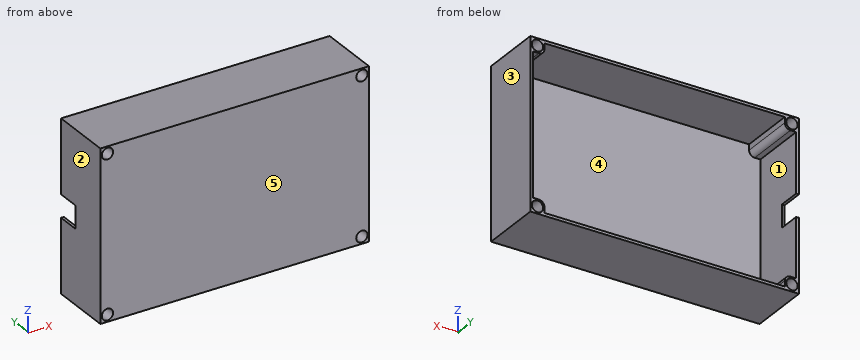
Autodesk Inventor part; units mm, degrees
ref_plane "YZ Plane" through (0, 0, 0) normal (1, 0, 0) x (0, 1, 0)
ref_plane "XZ Plane" through (0, 0, 0) normal (0, 1, 0) x (-1, 0, 0)
ref_plane "XY Plane" through (0, 0, 0) normal (0, 0, 1) x (1, 0, 0)
sketch "Szkic1" plane through (0, 0, 0) normal (0, 1, 0) x (-1, 0, 0)
  line L0 (0, 0) -> (90, 0)
  line L1 (90, 0) -> (90, -60)
  line L2 (90, -60) -> (0, -60)
  line L3 (0, -60) -> (0, 0)
  dimension "d0" = 90
  dimension "d1" = 60
extrude "Wyciągnięcie proste1" add sketch "Szkic1" along normal blind 2
sketch "Szkic15" plane through (-90, 0, -60) normal (-1, 0, 0) x (0, 0, 1)
  line L0 (0, 0) -> (60, 0)
  line L1 (60, 0) -> (60, 2)
  line L2 (60, 2) -> (0, 2)
  line L3 (0, 2) -> (0, 0)
extrude "Wyciągnięcie proste5" add sketch "Szkic15" along normal blind 5
sketch "Szkic16" plane through (0, 2, 0) normal (0, 1, 0) x (1, 0, 0)
  line L0 (0, 60) -> (-95, 60)
  line L1 (-95, 60) -> (-95, 0)
  line L2 (-94, 60) -> (-95, 60)
  line L3 (-95, 60) -> (-95, 0)
  line L4 (-95, 0) -> (-94, 0)
  line L5 (-94, 0) -> (-94, 60)
  line L6 (-95, 1) -> (0, 1)
  line L7 (0, 1) -> (0, 0)
  line L8 (0, 0) -> (-95, 0)
  line L9 (-95, 0) -> (-95, 1)
  line L10 (-1, 0) -> (0, 0)
  line L11 (0, 0) -> (0, 60)
  line L12 (0, 60) -> (-1, 60)
  line L13 (-1, 60) -> (-1, 0)
  line L14 (-1, 59) -> (-95, 59)
  line L15 (-95, 59) -> (-95, 60)
  line L16 (-95, 60) -> (-1, 60)
  line L17 (-1, 60) -> (-1, 59)
  point P0 (-94, 59)
  point P1 (-1, 1)
  point P2 (-94, 1)
extrude "Wyciągnięcie proste6" add sketch "Szkic16" along normal blind 20 contours L11 L6 L13 L0 | L13 L14 L5 L0 | L7 L8 L13 L6 | L5 L14 L1 L0 | L13 L8 L5 L6 | L5 L6 L1 L14 | L5 L4 L1 L6
sketch "Szkic21" plane through (0, 2, 0) normal (0, 1, 0) x (1, 0, 0)
  line L0 (-1, 59) -> (-1, 1)
  line L1 (-94, 1) -> (-1, 1)
  line L2 (-1, 5) -> (-5, 5)
  line L3 (-5, 5) -> (-5, 1)
  line L4 (-5, 1) -> (-1, 1)
  line L5 (-1, 1) -> (-1, 5)
  point P0 (0, 0)
  dimension "d61" = 4
extrude "Wyciągnięcie proste8" add sketch "Szkic21" along normal blind 20
sketch "Szkic22" plane through (0, 2, 0) normal (0, 1, 0) x (1, 0, 0)
  line L0 (-1, 59) -> (-1, 1)
  line L1 (-1, 55) -> (-5, 55)
  line L2 (-5, 55) -> (-5, 59)
  line L3 (-5, 59) -> (-1, 59)
  line L4 (-1, 59) -> (-1, 55)
  line L5 (-94, 1) -> (-94, 59)
  line L6 (-1, 59) -> (-94, 59)
  line L7 (-94, 55) -> (-90, 55)
  line L8 (-90, 55) -> (-90, 59)
  line L9 (-90, 59) -> (-94, 59)
  line L10 (-94, 59) -> (-94, 55)
  line L11 (-94, 1) -> (-5, 1)
  line L12 (-94, 5) -> (-90, 5)
  line L13 (-90, 5) -> (-90, 1)
  line L14 (-90, 1) -> (-94, 1)
  line L15 (-94, 1) -> (-94, 5)
  point P0 (0, 0)
  point P1 (-1, 5)
  dimension "d64" = 4
  dimension "d65" = 4
extrude "Wyciągnięcie proste9" add sketch "Szkic22" along normal blind 20
fillet "Zaokrąglenie1" radius 2 4 edges at (-90, 12, -55) (-5, 12, -55) (-90, 12, -5) (-5, 12, -5)
sketch "Szkic23" plane through (0, 22, 0) normal (0, 1, 0) x (1, 0, 0)
  point P0 (0, 0)
  point P1 (-2.5, 2.5)
  point P2 (-92.5, 2.5)
  point P3 (-92.5, 57.5)
  point P4 (-2.5, 57.5)
hole "Otwór5" at (-2.5, 22, -2.5) at (-92.5, 22, -2.5) at (-92.5, 22, -57.5) at (-2.5, 22, -57.5) direction (0, -1, 0) diameter 4 end through all
sketch "Szkic24" plane through (-95, 0, -60) normal (-1, 0, 0) x (0, 0, 1)
  point P0 (60, 0)
sketch "Szkic25" plane through (-95, 0, 0) normal (0, 0, 1) x (1, 0, 0)
  point P0 (95, 0)
sketch "Szkic26" plane through (-95, 0, -60) normal (-1, 0, 0) x (0, 0, 1)
  line L0 (60, 22) -> (0, 22)
  line L1 (26, 22) -> (34, 22)
  line L2 (34, 22) -> (34, 14)
  line L3 (34, 14) -> (26, 14)
  line L4 (26, 14) -> (26, 22)
  point P0 (60, 0)
  dimension "d76" = 8
  dimension "d77" = 8
extrude "Wyciągnięcie proste10" cut sketch "Szkic26" against normal blind 10
properties part number "góra"
Geometry: final body of the model. Coordinates: model frame, mm. Face numbers are marked on the shaded views. A direction names the side the tool comes from. Round coordinates to 2 decimals unless told otherwise and drop trailing zeros. Loops run counter-clockwise (first coordinate to the right, second up) from the corner with the lowest first, then second, coordinate; pieces in that order, holes last. Notation, with made-up numbers: (80, -12) -> (131, -12) arc R30 ccw to (131, 11) -> close; hole circle Ø3 at (-21, 57.5). An arc over 180 degrees is marked (long way). Write each question's results on one line, items separated by ' | '.
Item 1: Set-up query: the marked faces 1 and 2. Return all of +Z, -Z, +X, -X, +Y, -Y with unobstructed straight access to the full face (end or side cutting, diameter ignored); none if empty.
Answers below:
face 1: +Y | face 2: +Z, -Z, -X, +Y, -Y
Item 2: Cut plane B-B on y = 3. Return the cut outline in (x, z).
Answers below:
outline: (-95, -60) -> (0, -60) -> (0, 0) -> (-95, 0) -> close; hole circle Ø4 at (-92.5, -57.5); hole circle Ø4 at (-92.5, -2.5); hole (-94, -55) -> (-92, -55) arc R2 cw to (-90, -57) -> (-90, -59) -> (-5, -59) -> (-5, -57) arc R2 cw to (-3, -55) -> (-1, -55) -> (-1, -5) -> (-3, -5) arc R2 cw to (-5, -3) -> (-5, -1) -> (-90, -1) -> (-90, -3) arc R2 cw to (-92, -5) -> (-94, -5) -> close; hole circle Ø4 at (-2.5, -57.5); hole circle Ø4 at (-2.5, -2.5)
Item 3: Cut plane C-C on x = -42.5. Return the cut outline in (y, z), and give its area (3 significant figures).
Answers below:
outline: (0, -60) -> (22, -60) -> (22, -59) -> (2, -59) -> (2, -1) -> (22, -1) -> (22, 0) -> (0, 0) -> close | area: 160 mm²
Item 4: Pin query (flat end, axial travel): pin 1 Ø5 at (x, z) = (-64, -43.5) entering from +Y. Return the tip coordinate at first contact, or that it passes through.
Answers below:
pin 1: stops at y = 2
Item 5: Cut plane A-A on z = -51. Return the cut outline in (x, y).
Answers below:
outline: (-95, 0) -> (0, 0) -> (0, 22) -> (-1, 22) -> (-1, 2) -> (-94, 2) -> (-94, 22) -> (-95, 22) -> close
Item 6: Pull-direction query (X, two-part tool) for the marked faces 3, 4 and 5; classes: pulls with the +X half, pulls with the -X half, needs draft (parallel to the pull), parting line crosses it, or undercut.
Answers below:
face 3: pulls with the +X half | face 4: undercut | face 5: needs draft
Item 7: Line query: probe 1 along Z at (x, y) = (-92.5, 12.75); probe 2 along X at (y, z) = (16.5, -2.5); probe 3 along X at (y, z) = (7.5, -9). Output: solid intervals per line, ascending. Write a range as [from, to].
Answers below:
probe 1: z = [-60, -59.5], [-55.5, -55], [-5, -4.5], [-0.5, 0] | probe 2: x = [-95, -94.5], [-90.5, -90], [-5, -4.5], [-0.5, 0] | probe 3: x = [-95, -94], [-1, 0]
